from build123d import *

# Parameters (mm, degrees)
SKETCH1_W             = 41.275
SKETCH1_H             = 20.6375
BASE_FLANGE1_DEPTH    = 4.7625
BREAK_CORNER1_DEPTH   = 4.7625
M6X1_0_TAPPED_HOLE1_D = 5


# Read off the part's stored shape, not the designer's step: Break-Corner1
# Sheet-metal steps are written as plain solids
with BuildPart() as part:
    # Sketch1 → Base-Flange1 (new body)
    with BuildSketch(Plane.XY):
        Rectangle(SKETCH1_W, SKETCH1_H)
    extrude(amount=BASE_FLANGE1_DEPTH)

    # Break-Corner1 outline → Break-Corner1 (cut)
    with BuildSketch(Plane.XY):
        with BuildLine():
            Line((-20.6375, 10.31875), (-20.6375, 3.96875))
            ThreePointArc((-20.6375, 3.96875), (-18.777628061, 8.458878061), (-14.2875, 10.31875))
            Line((-14.2875, 10.31875), (-20.6375, 10.31875))
        make_face()
        with BuildLine():
            ThreePointArc((-14.2875, -10.31875), (-18.777628061, -8.458878061), (-20.6375, -3.96875))
            Line((-20.6375, -3.96875), (-20.6375, -10.31875))
            Line((-20.6375, -10.31875), (-14.2875, -10.31875))
        make_face()
        with BuildLine():
            Line((20.6375, 10.31875), (14.2875, 10.31875))
            ThreePointArc((14.2875, 10.31875), (18.777628061, 8.458878061), (20.6375, 3.96875))
            Line((20.6375, 3.96875), (20.6375, 10.31875))
        make_face()
        with BuildLine():
            ThreePointArc((20.6375, -3.96875), (18.777628061, -8.458878061), (14.2875, -10.31875))
            Line((14.2875, -10.31875), (20.6375, -10.31875))
            Line((20.6375, -10.31875), (20.6375, -3.96875))
        make_face()
    extrude(amount=BREAK_CORNER1_DEPTH, mode=Mode.SUBTRACT)

    # M6x1.0 Tapped Hole1 (through all)
    with Locations(Plane.XY.offset(4.7625)):
        with Locations((-12.7, 2.38125), (12.7, 2.38125)):
            Hole(M6X1_0_TAPPED_HOLE1_D / 2)


solid = part.part
Model file for the job. Use its own axes, mm. Give positions to 0.01 mm unless a question says otherwise; leave off trailing zeros. Order: outer loops, then holes, each group sorted by start corner. A loop starts at its lowest first (then second) coordinate and runs counter-clockwise, first axis right, second up. Notation, with made-up numbers: M 57,2.25 L 89,2.25 A16 cw 89,29.25 Z; hole C 88,79 d6. An arc over 180 degrees is marked long. Put each result on its own line as item: value. Start each with the question number.
(1) Band-saw the part on C-C on y = 7.75. Give the cut face in (x, z), then the cut area to 3 significant figures.
(2) Drill centre lines: L1, parallel to X at y = 2.5, z = 1.2; L2, parallel to Y at x = 12.7, z = 1.7; L3, parallel to X at y = 1.5, z = 2.1. Where is each one in solid material? Low to high. Write a range as [from, to].
(3) Band-saw the part on A-A on x = -12.7. Give the cut face in (y, z).
(4) Band-saw the part on B-B on z = 2.4. Give the cut face in (x, y).
(5) Pull direction X, two halves, no side cores. Call faces 1 (the face through (0, -10.319, 2)), 2 (the face through (-15.085, 3.132, 2.348)), 3 (the face through (18.827, -8.409, 2.348)), 4 (the face through (15.198, 2.491, 2.348)): released by +X, released by -X, zero draft, split by the parting line, or undercut.
Results below:
1. outline: M -19.39,0 L 19.39,0 L 19.39,4.76 L -19.39,4.76 Z
1. area: 185 mm2
2. L1: x = [-20.64, -15.2], [-10.2, 10.2], [15.2, 20.64]
2. L2: y = [-10.32, -0.12], [4.88, 10.32]
2. L3: x = [-20.64, -15.04], [-10.36, 10.36], [15.04, 20.64]
3. outline: M -10.32,0 L -0.12,0 L -0.12,4.76 L -10.32,4.76 Z; M 4.88,0 L 10.32,0 L 10.32,4.76 L 4.88,4.76 Z
4. outline: M -20.64,-3.97 A6.35 ccw -14.29,-10.32 L 14.29,-10.32 A6.35 ccw 20.64,-3.97 L 20.64,3.97 A6.35 ccw 14.29,10.32 L -14.29,10.32 A6.35 ccw -20.64,3.97 Z; hole C -12.7,2.38 d5; hole C 12.7,2.38 d5
5. face 1: zero draft
5. face 2: undercut
5. face 3: released by +X
5. face 4: undercut
